The drawing under review shows one solid part. Ordinate dimensions are in mm from its lowest x, y, z. Give positions to 0.01 mm unless a question says otherwise; leave off trailing zeros. Order: outer loops, then holes, each group sorted by start corner. A loop starts at its lowest first (then second) coordinate and runs counter-clockwise, first axis right, second up. Notation, with made-up numbers: (39.5, -24) - (87.5, -24) arc R31 ccw to (87.5, 11) - close; hole circle Ø11 at (31.5, 88). An arc over 180 degrees is marked (long way). Write item = value, one per line. Start each with the question number.
1. Wall thickness on probe 1 along Z at (x, y) = (65, 0.55); probe 2 along X at (y, z) = (1.5, 65); probe 3 along Z at (x, y) = (66, 2.6) (1 decimal): over which ranges is each line inside the solid? List them lowest first.
2. For P1, Ø2.5, axis at x = 10, z = 74.5, coming from the +Y side; P2, Ø2.5, axis at x = 3, y = 3.5, coming from the -Z side; P3, Ø4, axis at x = 64.95, z = 7.5, coming from the -Y side; P4, Ø1, axis at x = 112.5, y = 2, coming from the +Z side, all flat-tipped, find the tip position at first contact; note any pin that passes through.
3. We need section C-C, the plane y = 1.65. State how many separate pieces and enclosed holes the cut face has, and give its area (3 significant figures).
4. We need section B-B, the plane x = 53. Give the boundary of the cut face in (y, z).
5. We need section A-A, the plane z = 65. Give the boundary of the cut face in (x, y).
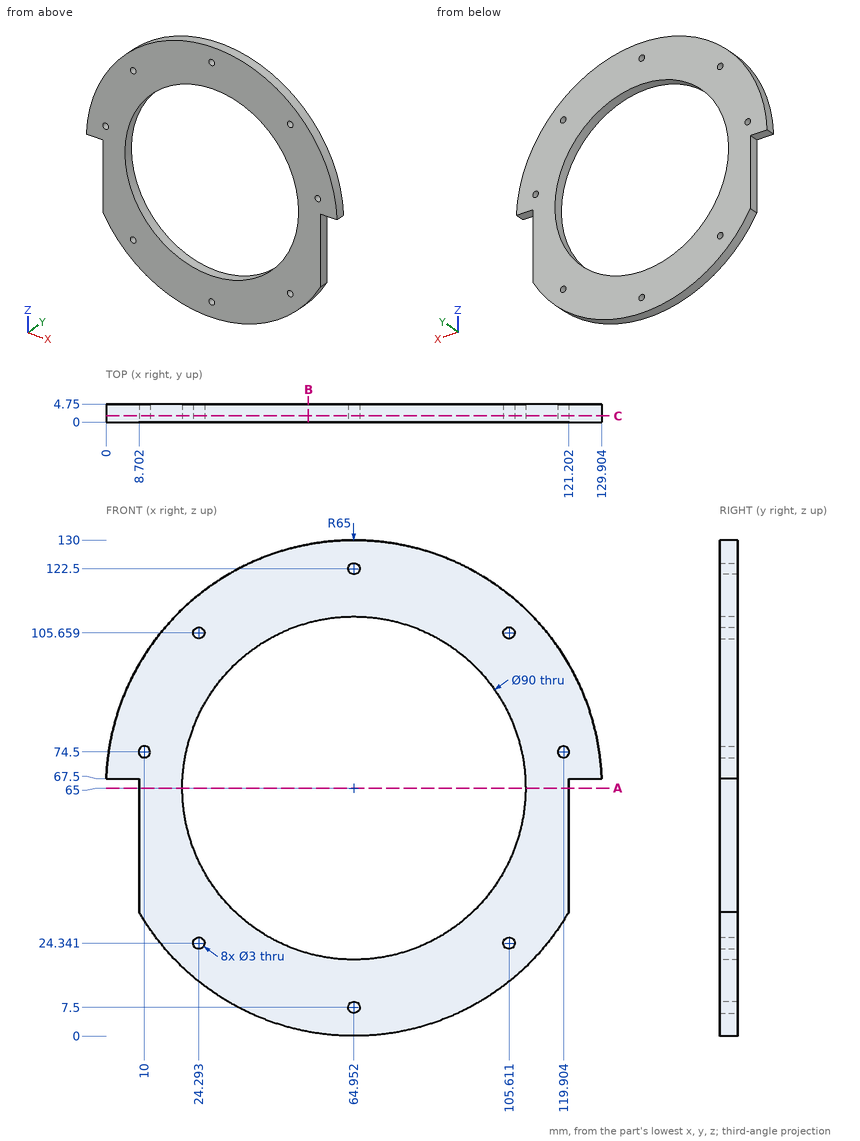
Model answer:
q1.probe_1 = 0 to 6, 9 to 20, 110 to 121, 124 to 130
q1.probe_2 = 8.7 to 19.95, 109.95 to 121.2
q1.probe_3 = 0 to 6.4, 8.6 to 20, 110 to 121.4, 123.6 to 130
q2.P1 = through
q2.P2 = 67.5
q2.P3 = 0
q2.P4 = 109.85
q3.separate_pieces = 1
q3.enclosed_holes = 9
q3.area = 6,430 mm2
q4.outline = (0, 1.11) - (4.75, 1.11) - (4.75, 21.62) - (0, 21.62) - close; (0, 108.38) - (4.75, 108.38) - (4.75, 128.89) - (0, 128.89) - close
q5.outline = (8.7, 0) - (19.95, 0) - (19.95, 4.75) - (8.7, 4.75) - close; (109.95, 0) - (121.2, 0) - (121.2, 4.75) - (109.95, 4.75) - close
